Model file for the job. Use its own axes, mm. A direction names the side the tool comes from. Coordinates: 2 decimals unless noted, no trailing zeros. Loops run counter-clockwise (first coordinate to the right, second up) from the corner with the lowest first, then second, coordinate; pieces in that order, holes last.
from build123d import *

# Parameters (mm, degrees)
F1_DEPTH = 30.5
F2_DEPTH = 25.5


with BuildPart() as f1:
    # F0 (on Top) → F1 (new body)
    with BuildSketch(Plane.XY):
        Polygon((10.524174, 6.35), (-3.666174, 6.35), (-10.761348, -5.939202), (-3.666174, -18.228404), (10.524174, -18.228404), (17.619348, -5.939202), align=None)
        Polygon((-3.429, -5.939202), (0, 0), (6.858, 0), (10.287, -5.939202), (6.858, -11.878404), (0, -11.878404), align=None, mode=Mode.SUBTRACT)
    extrude(amount=F1_DEPTH)

    # F0 (on Top) → F2 (join)
    with BuildSketch(Plane.XY):
        Polygon((17.619348, -18.228404), (17.619348, -5.939202), (10.524174, -18.228404), align=None)
        Polygon((-10.761348, -5.939202), (-3.666174, 6.35), (-10.761348, 6.35), align=None)
    extrude(amount=F2_DEPTH)


solid = f1.part
Q1. Flat gauge pins, fed straight in: P1, Ø3, axis at y = -2.5, z = 6, coming from the +X side; P2, Ø3, axis at y = 3.5, z = 19.5, coming from the +X side. Where does each tip first touch, or does it go through?
Answers:
P1: stops at x = 16.5
P2: stops at x = 13.04
Q2. Mould opens along X. For faces 1 (the flat face through (-1.74, -3.01, 15.04)), 2 (the flat face through (-7.164, 0.291, 27.965)), 3 (the flat face through (-8, 2, 25.5)) say: +X half, -X half, draft (parallel to the pull), parting line (faces both ways), or undercut.
Answers:
face 1: undercut
face 2: -X half
face 3: draft
Q3. Slice it at A-A (z = 23.5). List the corners of the cut face in (x, y).
Answers:
outline: (-10.76, -5.94) - (-3.67, -18.23) - (17.62, -18.23) - (17.62, -5.94) - (10.52, 6.35) - (-10.76, 6.35) - close; hole (-3.43, -5.94) - (0, -11.88) - (6.86, -11.88) - (10.29, -5.94) - (6.86, 0) - (0, 0) - close
Q4. Slice it at C-C (y = -2.25). List the corners of the cut face in (x, z).
Answers:
outline: (-10.76, 0) - (-1.3, 0) - (-1.3, 30.5) - (-8.63, 30.5) - (-8.63, 25.5) - (-10.76, 25.5) - close; (8.16, 0) - (15.49, 0) - (15.49, 30.5) - (8.16, 30.5) - close
Q5. Drill centre lines: line 1 (Y direction, x = 2, z = 11.5); line 2 (X direction, y = -8.5, z = 9.5); line 3 (Y direction, x = 9, z = 10.5). Where is each one in solid material? Low to high.
Answers:
line 1: y = -18.23 to -11.88, 0 to 6.35
line 2: x = -9.28 to -1.95, 8.81 to 17.62
line 3: y = -18.23 to -8.17, -3.71 to 6.35
Q6. Which spindle directions (+Z, -Z, +X, -X, +Y, -Y) get a long thin tool onto all of the face, cutting with end or side? Do faces 4 (the flat face through (8.597, -8.867, 15.036)), 5 (the flat face through (14.02, -12.17, 27.96)), 6 (the flat face through (7, -18.228, 15)). Say none if no direction does.
Answers:
face 4: +Z, -Z
face 5: +Z, +X, -Y
face 6: +Z, -Z, +X, -X, -Y
Q7. Slice it at B-B (x = 6.25). List the corners of the cut face in (y, z).
Answers:
outline: (-18.23, 0) - (-11.88, 0) - (-11.88, 30.5) - (-18.23, 30.5) - close; (0, 0) - (6.35, 0) - (6.35, 30.5) - (0, 30.5) - close
Q8. Slice it at D-D (z = 28.5). List the corners of the cut face in (x, y).
Answers:
outline: (-10.76, -5.94) - (-3.67, -18.23) - (10.52, -18.23) - (17.62, -5.94) - (10.52, 6.35) - (-3.67, 6.35) - close; hole (-3.43, -5.94) - (0, -11.88) - (6.86, -11.88) - (10.29, -5.94) - (6.86, 0) - (0, 0) - close
